from build123d import *

# Parameters (mm, degrees)
SKETCH2_R               = 10
BOSS_EXTRUDE1_DEPTH     = 40
SKETCH3_W               = 4
SKETCH3_H               = 30
CUT_EXTRUDE1_DEPTH      = 20
CUT_EXTRUDE1_DEPTH_BACK = 20
SKETCH4_R               = 4
CUT_EXTRUDE2_DEPTH      = 20
CUT_EXTRUDE2_DEPTH_BACK = 20
SKETCH5_R               = 5
BOSS_EXTRUDE2_DEPTH     = 90
SKETCH6_R               = 3.8
CUT_EXTRUDE3_DEPTH      = 20


with BuildPart() as part:
    # Sketch2 → Boss-Extrude1 (new body)
    with BuildSketch(Plane.XY):
        Circle(SKETCH2_R)
    extrude(amount=BOSS_EXTRUDE1_DEPTH)

    # Sketch3 → Cut-Extrude1 (cut, two sides)
    with BuildSketch(Plane(origin=(0, 0, 0), x_dir=(1, 0, 0), z_dir=(0, 1, 0))) as cut_extrude1_sk:
        with Locations((0, -15)):
            Rectangle(SKETCH3_W, SKETCH3_H)
    extrude(amount=CUT_EXTRUDE1_DEPTH, mode=Mode.SUBTRACT)
    extrude(cut_extrude1_sk.sketch, amount=-CUT_EXTRUDE1_DEPTH_BACK, mode=Mode.SUBTRACT)

    # Sketch4 → Cut-Extrude2 (cut, two sides)
    with BuildSketch(Plane(origin=(0, 0, 0), x_dir=(0, 0, -1), z_dir=(1, 0, 0))) as cut_extrude2_sk:
        with Locations((-7, 0)):
            Circle(SKETCH4_R)
    extrude(amount=CUT_EXTRUDE2_DEPTH, mode=Mode.SUBTRACT)
    extrude(cut_extrude2_sk.sketch, amount=-CUT_EXTRUDE2_DEPTH_BACK, mode=Mode.SUBTRACT)

    # Sketch5 → Boss-Extrude2 (add)
    with BuildSketch(Plane.XY.offset(40)):
        Circle(SKETCH5_R)
    extrude(amount=BOSS_EXTRUDE2_DEPTH)

    # Sketch6 → Cut-Extrude3 (cut)
    with BuildSketch(Plane.XY.offset(130)):
        Circle(SKETCH6_R)
    extrude(amount=-CUT_EXTRUDE3_DEPTH, mode=Mode.SUBTRACT)


solid = part.part
Model file for the job. Use its own axes, mm. A direction names the side the tool comes from. Coordinates: 2 decimals unless noted, no trailing zeros. Order: outer loops, then holes, each group sorted by start corner. A loop starts at its lowest first (then second) coordinate and runs counter-clockwise, first axis right, second up. Notation, with made-up numbers: M 29,-9 L 54,-9 A13 ccw 54,9 Z; hole C 78.25,21.5 d4. An arc over 180 degrees is marked long. Return JSON: item names as keys, results as strings.
1. Saw through at D-D (x = -6.75). Give the cut face in (y, z).
Ans:
{"outline": "M -7.38,0 L 7.38,0 L 7.38,40 L -7.38,40 Z; hole C 0,7 d8"}
2. Drill centre lines: probe 1 along Z at (x, y) = (5.5, 0); probe 2 along Y at (x, z) = (0, 123.25); probe 3 along Z at (x, y) = (-0.75, 9). Where is each one in solid material? Low to high.
Ans:
{"probe 1": "0 to 3, 11 to 40", "probe 2": "-5 to -3.8, 3.8 to 5", "probe 3": "30 to 40"}
3. Tool access for faces 1 (the face through (-5, 0, 0)), 2 (the face through (0, 0, 110)), 3 (the face through (0, 0, 30)): list every direction of +Z, -Z, +X, -X, +Y, -Y with a clear straight run to the whole face (end or side of a thin tool).
Ans:
{"face 1": "-Z, +X, -X, +Y, -Y", "face 2": "+Z", "face 3": "-Z, +Y, -Y"}
4. Pull direction Y, two halves, no side cores. Call faces 4 (the face through (-6, 0, 11)), 5 (the face through (-1, 4, 130)), 6 (the face through (4.614, -8.872, 19.72)): +Y half, -Y half, draft (parallel to the pull), parting line (faces both ways), or undercut.
Ans:
{"face 4": "undercut", "face 5": "draft", "face 6": "parting line"}
5. Saw through at C-C (x = 0). Give the cut face in (y, z), and give its area (3 significant figures).
Ans:
{"outline": "M -10,30 L 10,30 L 10,40 L 5,40 L 5,130 L 3.8,130 L 3.8,110 L -3.8,110 L -3.8,130 L -5,130 L -5,40 L -10,40 Z", "area": "948 mm^2"}
6. Saw through at A-A (y = 0). Give the cut face in (x, z), and give its area (3 significant figures).
Ans:
{"outline": "M -10,0 L -2,0 L -2,3 L -10,3 Z; M -10,11 L -2,11 L -2,30 L 2,30 L 2,11 L 10,11 L 10,40 L 5,40 L 5,130 L 3.8,130 L 3.8,110 L -3.8,110 L -3.8,130 L -5,130 L -5,40 L -10,40 Z; M 2,0 L 10,0 L 10,3 L 2,3 Z", "area": "1,300 mm^2"}
7. Saw through at B-B (z = 7). Give the cut face in (x, y), and give its area (3 significant figures).
Ans:
{"outline": "M -9.17,-4 A10 ccw -2,-9.8 L -2,-4 Z; M -9.17,4 L -2,4 L -2,9.8 A10 ccw Z; M 2,-9.8 A10 ccw 9.17,-4 L 2,-4 Z; M 2,4 L 9.17,4 A10 ccw 2,9.8 Z", "area": "111 mm^2"}
8. Flat gauge pins, fed straight in: pin 1 (4 mm diameter, centred on y = -7.5, z = 40.5, fed in from -X); pin 2 (8 mm diameter, centred on y = -6.5, z = 40, fed in from +X); pin 3 (6 mm diameter, centred on x = 5.5, z = 46.5, fed in from +Y). Where does each tip first touch, or does it go through?
Ans:
{"pin 1": "x = -8.31", "pin 2": "x = 9.68", "pin 3": "y = 4.33"}
